Design review of the part built by this model. Coordinates are the model's own, in mm. Coordinates: 2 decimals unless noted, no trailing zeros. Write each loop counter-clockwise with the first axis right and the second up, starting at its lowest first coordinate (ties: lowest second). Pieces come first, ordered by that corner, then holes. Notation, with made-up numbers: (-34.75, -36) - (-9.75, -36) arc R28 cw to (-9.75, -5) - close; hole circle Ø7 at (-24, 67). An arc over 180 degrees is marked (long way). Use a Markdown table: item, result.
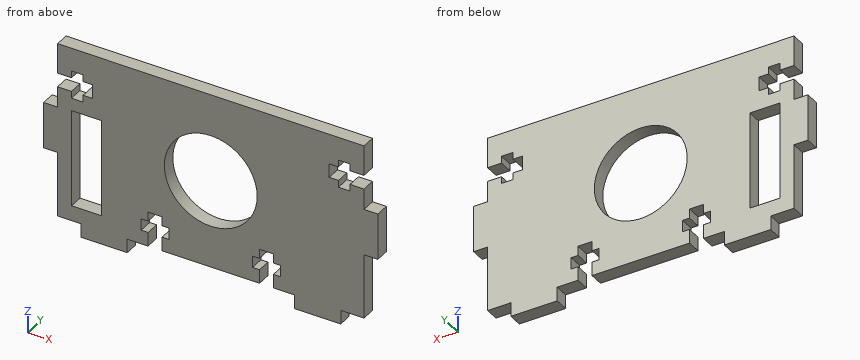
from build123d import *

# Parameters (mm, degrees)
F0_W     = 6.5
F0_H     = 21
F0_R     = 10
F1_DEPTH = 3
F3_DEPTH = 3


# Not quite as in the source:
# - a feature names something its author has since deleted; it is built from what else it names


with BuildPart() as f1:
    # F0 (on Front) → F1 (new body)
    with BuildSketch(Plane.XZ):
        Polygon((33, 5), (33, 19), (-33, 19), (-33, 5), (-36, 5), (-36, -5), (-33, -5), (-33, -19), (-28, -19), (-28, -22), (-18, -22), (-18, -19), (0, -19), (18, -19), (18, -22), (28, -22), (28, -19), (33, -19), (33, -5), (36, -5), (36, 5), align=None)
        with Locations((-26.75, -5.25)):
            Rectangle(F0_W, F0_H, mode=Mode.SUBTRACT)
        Circle(F0_R, mode=Mode.SUBTRACT)
    extrude(amount=F1_DEPTH)

    # F2 (on face) → F3 (cut, through all)
    with BuildSketch(Plane.XZ.offset(3)):
        Polygon((10.5, -16), (10.5, -19), (13.5, -19), (13.5, -16), (15, -16), (15, -13.5), (13.5, -13.5), (13.5, -11.5), (10.5, -11.5), (10.5, -13.5), (9, -13.5), (9, -16), align=None)
        Polygon((30, 9.5), (33, 9.5), (33, 12.5), (30, 12.5), (30, 14), (27.5, 14), (27.5, 12.5), (25.5, 12.5), (25.5, 9.5), (27.5, 9.5), (27.5, 8), (30, 8), align=None)
        Polygon((-33, 12.5), (-33, 9.5), (-30, 9.5), (-30, 8), (-27.5, 8), (-27.5, 9.5), (-25.5, 9.5), (-25.5, 12.5), (-27.5, 12.5), (-27.5, 14), (-30, 14), (-30, 12.5), align=None)
        Polygon((-13.5, -19), (-10.5, -19), (-10.5, -16), (-9, -16), (-9, -13.5), (-10.5, -13.5), (-10.5, -11.5), (-13.5, -11.5), (-13.5, -13.5), (-15, -13.5), (-15, -16), (-13.5, -16), align=None)
    extrude(amount=-F3_DEPTH, mode=Mode.SUBTRACT)


solid = f1.part
(1) Take a section at D-D on x = 8. Write out the cut boundary in (y, z), and give its area (3 significant figures).
Determined:
| item | result |
|---|---|
| outline | (-3, -19) - (0, -19) - (0, -6) - (-3, -6) - close; (-3, 6) - (0, 6) - (0, 19) - (-3, 19) - close |
| area | 78.0 mm2 |
(2) For pin 1 (0.8 mm diameter, centred on x = 29, y = -1.5, fed in from -Z); pin 2 (1.2 mm diameter, centred on y = -1.5, z = 13.5, fed in from +X); pin 3 (1.2 mm diameter, centred on y = -2, z = 13, fed in from -X), all flat-tipped, find the tip position at first contact; note any pin that passes through.
Determined:
| item | result |
|---|---|
| pin 1 | z = -19 |
| pin 2 | x = 33 |
| pin 3 | x = -33 |
(3) Take a section at B-B on x = -26.5. Write out the cut boundary in (y, z), and give its area (3 significant figures).
Determined:
| item | result |
|---|---|
| outline | (-3, -22) - (0, -22) - (0, -15.75) - (-3, -15.75) - close; (-3, 5.25) - (0, 5.25) - (0, 9.5) - (-3, 9.5) - close; (-3, 12.5) - (0, 12.5) - (0, 19) - (-3, 19) - close |
| area | 51.0 mm2 |
(4) Take a section at A-A on z = 0. Write out the cut boundary in (x, y), and give its area (4 significant figures).
Determined:
| item | result |
|---|---|
| outline | (-36, -3) - (-30, -3) - (-30, 0) - (-36, 0) - close; (-23.5, -3) - (-10, -3) - (-10, 0) - (-23.5, 0) - close; (10, -3) - (36, -3) - (36, 0) - (10, 0) - close |
| area | 136.5 mm2 |
(5) For L1, parallel to X at y = -1, z = -14; L2, parallel to X at y = -2.35, z = -20; L3, parallel to X at y = -2.8, z = 2.5, list the stretches that pass through material, from the lowest coordinate up. Write a range as from..to.
Determined:
| item | result |
|---|---|
| L1 | -33..-30, -23.5..-15, -9..9, 15..33 |
| L2 | -28..-18, 18..28 |
| L3 | -36..-30, -23.5..-9.68, 9.68..36 |
(6) Take a section at C-C on z = 6. Write out the cut boundary in (x, y).
Determined:
| item | result |
|---|---|
| outline | (-33, -3) - (-8, -3) - (-8, 0) - (-33, 0) - close; (8, -3) - (33, -3) - (33, 0) - (8, 0) - close |
